from build123d import *

# Parameters (mm, degrees)
F0_W     = 123.5685497522
F0_H     = 125.5645230412
F1_DEPTH = 100
F3_DEPTH = 25
F4_R     = 5


with BuildPart() as f1:
    # F0 (on Top) → F1 (new body)
    with BuildSketch(Plane.XY):
        with Locations((2.0866915584, 3.2661296427)):
            Rectangle(F0_W, F0_H)
    extrude(amount=F1_DEPTH)

    # F2 (on face) → F3 (cut)
    with BuildSketch(Plane.XZ.offset(59.5161318779)):
        Polygon((0, 75.206823647), (-30.6101683527, 26.9990302622), (33.7249785662, 26.9990302622), align=None)
    extrude(amount=-F3_DEPTH, mode=Mode.SUBTRACT)

    # F4
    f4_edges = [f1.edges().sort_by_distance(p)[0] for p in [
        (0, -47.016132, 75.206824),
        (-30.610168, -47.016132, 26.99903),
        (33.724979, -47.016132, 26.99903),
    ]]
    fillet(f4_edges, radius=F4_R)


solid = f1.part
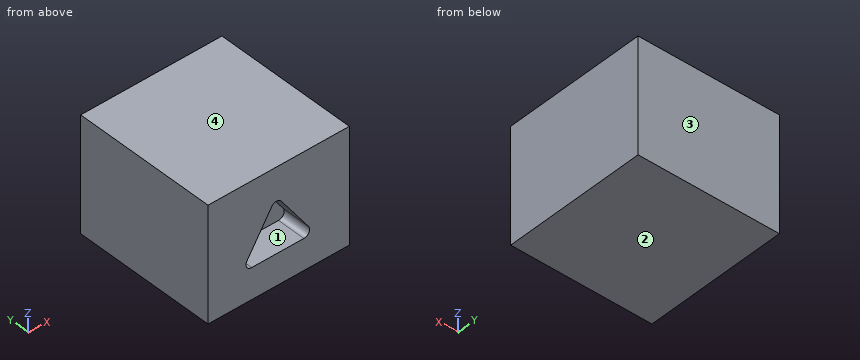
CAD build for the part. Positions are in the model's coordinates, mm. Face numbers are marked on the shaded views. Coordinates: 2 decimals unless noted, no trailing zeros. Write each loop counter-clockwise with the first axis right and the second up, starting at its lowest first coordinate (ties: lowest second). Pieces come first, ordered by that corner, then holes. Notation, with made-up numbers: M 15,73 L 33,73 A38 ccw 33,112 Z; hole C 5,-18 d6. An arc over 180 degrees is marked long. Answer as a JSON object with one key per item and string values. Group by question number.
1) Saw through at A-A (y = -42.5). Write the cut outline in (x, z), plus the area to 3 significant figures.
2) Wall check: line 1 (Y direction, x = -2.5, z = 27.5); line 2 (Z direction, x = 21.5, y = -41); line 3 (Z direction, x = -25, y = -38). Give the ranges that are in metal, low to high. Write a range as from..to.
3) Saw through at C-C (z = 59). Write the cut outline in (x, y).
4) Mould opens along Z. For the marked faces 1, 2, 3 and 4 say: +Z half, -Z half, draft (parallel to the pull), parting line (faces both ways), or undercut.
5) Saw through at B-B (x = 8.5). Write the cut outline in (y, z).
Values follow:
{
 "1": {"outline": "M -59.7,0 L 63.87,0 L 63.87,100 L -59.7,100 Z; hole M -25.73,34.68 A5 ccw -21.51,27 L 24.13,27 A5 ccw 28.22,34.87 L 4.3,69.06 A5 ccw -4.02,68.88 Z", "area": "10,900 mm2"},
 "2": {"line 1": "y = -34.52..66.05", "line 2": "z = 0..27, 44.47..100", "line 3": "z = 0..28.42, 35.83..100"},
 "3": {"outline": "M -59.7,-59.52 L -10.29,-59.52 L -10.29,-34.52 L 11.34,-34.52 L 11.34,-59.52 L 63.87,-59.52 L 63.87,66.05 L -59.7,66.05 Z"},
 "4": {"face 1": "undercut", "face 2": "-Z half", "face 3": "draft", "face 4": "+Z half"},
 "5": {"outline": "M -59.52,0 L 66.05,0 L 66.05,100 L -59.52,100 L -59.52,63.06 L -34.52,63.06 L -34.52,27 L -59.52,27 Z"}
}
